Check sheet for the modelled part. Datum: model origin and axes. Units: mm. Face numbers are marked on the shaded views. Give positions to 0.01 mm unless a question says otherwise; leave off trailing zeros. Loops run counter-clockwise (first coordinate to the right, second up) from the corner with the lowest first, then second, coordinate; pieces in that order, holes last. Notation, with made-up numbers: (-33.5, 28.5) -> (23.5, 28.5) arc R28 ccw to (23.5, 58.5) -> close; hole circle Ø1 at (-25, 81.5). An arc over 180 degrees is marked (long way). Answer as CSV lines item,"result". Start each with the question number.
(1) Material ranges on line 1 (X direction, y = 3.75, z = -0.25); line 2 (X direction, y = 0.75, z = 0.25); line 3 (Z direction, x = -0.5, y = -0.5), recorded low to high. Write a range as from..to.
(2) Section check B-B on x = 7.5. Enter the section's corners in (y, z), plus the area to 3 significant figures.
(3) Gauge pin test, flat ends, axial feed: pin 1 Ø4 at (x, y) = (2.5, 3) entering from -Z; pin 2 Ø0.8 at (x, z) = (-1.5, 0.5) entering from -Y; pin 3 Ø1.5 at (x, z) = (12.5, -1.5) entering from -Y; pin 4 Ø3 at (y, z) = (3, 0) entering from +X. Record the tip position at first contact, or that the pin passes through.
(4) Section check A-A on x = 0. Enter the section's corners in (y, z).
(5) Release check for a two-part mould opening along Y. For the marked faces 1, 2 and 3 record: pulls with the +Y half, pulls with the -Y half, needs draft (parallel to the pull), parting line crosses it, or undercut.
from build123d import *

# Parameters (mm, degrees)
SLOT_CUT_EXTRUDE1_DEPTH      = 17.90568942
SLOT_CUT_EXTRUDE1_DEPTH_BACK = 17.90568942
SKETCH2_W                    = 1
SKETCH2_H                    = 1.2
SKETCH11_W                   = 2.8
SKETCH11_H                   = 0.333333333
POINT_CUT_EXTRUDE8_DEPTH     = 17.90568942


with BuildPart() as part:
    # Sketch1 → base-Revolve (revolve)
    with BuildSketch(Plane.XY, mode=Mode.PRIVATE) as base_revolve_sk:
        with BuildLine():
            Line((0.238648539, 3.761351461), (2.165685425, 1.834314575))
            ThreePointArc((2.165685425, 1.834314575), (2.425224104, 1.660896374), (2.73137085, 1.6))
            Line((2.73137085, 1.6), (3.7, 1.6))
            Line((3.7, 1.6), (4.1, 2))
            Line((4.1, 2), (16, 2))
            Line((16, 2), (16, 0))
            Line((16, 0), (0, 0))
            Line((0, 0), (-1.730540111, 0))
            ThreePointArc((-1.730540111, 0), (-1.345987021, 2.01818082), (-0.246219246, 3.753532584))
            ThreePointArc((-0.246219246, 3.753532584), (-0.005441747, 3.860159049), (0.238648539, 3.761351461))
        make_face()
    revolve(base_revolve_sk.sketch.rotate(Axis((0, 0, 0), (1, 0, 0)), 90), axis=Axis((0, 0, 0), (1, 0, 0)))

    # Sketch2 → slot_Cut-Extrude1 (cut, two sides: drawn at the far end of the back side and taken through both)
    with BuildSketch(Plane.XY.offset(-SLOT_CUT_EXTRUDE1_DEPTH_BACK)):
        with Locations((-1.230540111, 0)):
            Rectangle(SKETCH2_W, SKETCH2_H)
    extrude(amount=SLOT_CUT_EXTRUDE1_DEPTH + SLOT_CUT_EXTRUDE1_DEPTH_BACK, mode=Mode.SUBTRACT)

    # Sketch8 → point_Cut-Revolve1 (revolve, cut)
    with BuildSketch(Plane.XY, mode=Mode.PRIVATE) as point_cut_revolve1_sk:
        Polygon((16, 0), (16.508, 0), (16.508, 2.508), (15.194596374, 2.508), (15.194596374, 2), (16, 1.535), align=None)
    revolve(point_cut_revolve1_sk.sketch.rotate(Axis((0, 0, 0), (1, 0, 0)), 90), axis=Axis((0, 0, 0), (1, 0, 0)), mode=Mode.SUBTRACT)

    # Sketch11 → point_Cut-Extrude8 (cut, through all)
    with BuildSketch(Plane.XY):
        with Locations((14.6, -0.166666667)):
            Rectangle(SKETCH11_W, SKETCH11_H)
    extrude(amount=POINT_CUT_EXTRUDE8_DEPTH, mode=Mode.SUBTRACT)


solid = part.part
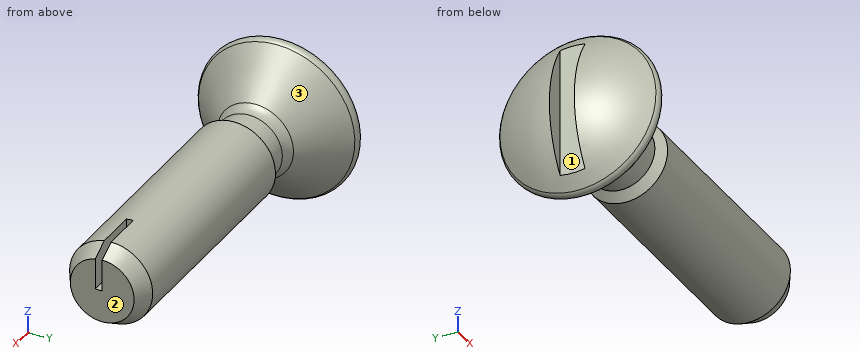
Working result:
1,line 1,"x = -0.24..0.24"
1,line 2,"x = -1.67..16"
1,line 3,"z = -3.43..3.43"
2,outline,"circle Ø4 at (0, 0)"
2,area,"12.6 mm^2"
3,pin 1,"stops at z = -2.54"
3,pin 2,"stops at y = -2.51"
3,pin 3,"stops at y = -1.85"
3,pin 4,"stops at x = 16"
4,outline,"circle Ø7.72 at (0, 0)"
5,face 1,"undercut"
5,face 2,"needs draft"
5,face 3,"parting line crosses it"
